Verification items for the finished model (mm, model axes). A direction names the side the tool comes from. Coordinates: 2 decimals unless noted, no trailing zeros. Write each loop counter-clockwise with the first axis right and the second up, starting at its lowest first coordinate (ties: lowest second). Pieces come first, ordered by that corner, then holes. Notation, with made-up numbers: (33, -20.75) - (77, -20.75) arc R20 cw to (77, 8.25) - close; hole circle Ø2 at (24, 40.5). An arc over 180 degrees is marked (long way). Use CSV: the item, a comma, the result in double quotes. Start each with the question number.
Autodesk Fusion 360 part; units mm, degrees
sketch "Sketch1" plane through (0, 0, 0) normal (0, 1, 0) x (1, 0, 0)
  line L0 (17.5, 25) -> (-17.5, 25)
  line L1 (-17.5, 25) -> (-17.5, -25)
  line L2 (-17.5, -25) -> (17.5, -25)
  line L3 (17.5, -25) -> (17.5, 25)
  line L4 (17.5, 25) -> (-17.5, -25) construction
  line L5 (-17.5, 25) -> (17.5, -25) construction
  line L6 (25, 17.5) -> (-25, 17.5)
  line L7 (-25, 17.5) -> (-25, -17.5)
  line L8 (-25, -17.5) -> (25, -17.5)
  line L9 (25, -17.5) -> (25, 17.5)
  line L10 (25, 17.5) -> (-25, -17.5) construction
  line L11 (-25, 17.5) -> (25, -17.5) construction
  circle A0 centre (0, 0) radius 7.6
  circle A1 centre (0, 0) radius 6.4
  circle A2 centre (0, 0) radius 12.5
  circle A3 centre (-20, 7.5) radius 1.5
  circle A4 centre (-20, -7.5) radius 1.5
  circle A5 centre (-7.5, -20) radius 1.5
  circle A6 centre (7.5, -20) radius 1.5
  circle A7 centre (20, -7.5) radius 1.5
  circle A8 centre (20, 7.5) radius 1.5
  circle A9 centre (7.5, 20) radius 1.5
  circle A10 centre (-7.5, 20) radius 1.5
  dimension "d1" = 50
  dimension "d2" = 35
  dimension "d3" = 50
  dimension "d4" = 35
  dimension "d5" = 15.2
  dimension "d6" = 12.8
  dimension "d7" = 25
  dimension "d8" = 3
  dimension "d9" = 3
  dimension "d10" = 10
  dimension "d11" = 10
  dimension "d12" = 5
  dimension "d13" = 5
  dimension "d15" = 360
extrude "Extrude1" add sketch "Sketch1" along normal blind 3 contours L0 L1 L3 L6 | L3 L6 L8 L9 | L1 L3 L6 L8 | L1 L6 L7 L8 | L1 L2 L3 L8 makes body 1
extrude "Extrude2" add sketch "Sketch1" along normal blind 10 separate body contours A0 makes body 2
extrude "Extrude3" add sketch "Sketch1" along normal blind 40 contours A1 | A2 bodies 1 2
sketch "Sketch2" plane through (0, 10, 0) normal (0, 1, 0) x (-1, 0, 0)
  circle A0 centre (0, 0) radius 6.4
  circle A1 centre (0, 0) radius 7.6
sketch "Sketch4" plane through (0, 0, 0) normal (0, 0, 1) x (1, 0, 0)
  circle A0 centre (0, 20) radius 1.5
  line L0 (0, 20) -> (0, 0)
  dimension "d22" = 3
  dimension "d23" = 20
extrude "Extrude4" cut sketch "Sketch4" against normal blind 30 bodies 1
extrude "Extrude5" cut sketch "Sketch4" along normal blind 30 bodies 1
sketch "Sketch6" plane through (0, 0, 0) normal (1, 0, 0) x (0, 0, -1)
  circle A0 centre (0, 30) radius 1.5
  line L0 (0, 30) -> (0, 0)
  dimension "d28" = 3
  dimension "d29" = 30
extrude "Extrude6" cut sketch "Sketch6" against normal blind 30 bodies 1
extrude "Extrude7" cut sketch "Sketch6" along normal blind 30 bodies 1
sketch "Sketch7" plane through (0, 0, 0) normal (0, 1, 0) x (1, 0, 0)
  circle A0 centre (0, 0) radius 1
  dimension "d34" = 2
extrude "Extrude8" cut sketch "Sketch7" along normal blind 10 bodies 1
Q1. Scan lines: line 1 along Z through (x, y) = (20, 1.1); line 2 along X through (y, z) = (1.55, 7.5). Record each from-to range of solid material in increasing order. Write a range as from..to.
Q2. Release check for a two-part mould opening along Z. For faces 1 (the cylindrical face through (-8.61, 1.48, 21.01)), 2 (the flat face through (-21, 1, -17.5)), 3 (the flat face through (-5.9, 3, -11.5)) record: released by +Z, released by -Z, zero draft, split by the parting line, or undercut.
Q3. Tool access check on faces 4 (the flat face through (-17.5, 1, 21)), 5 (the flat face through (0, 10, 0)), 6 (the cylindrical face through (6.104, 24.79, 1.922)), 7 (the flat face through (21, 1, -17.5)). Record the directions out of +Z, -Z, +X, -X, +Y, -Y that give a thin tool (end or side, any length) a straight path to the whole face; none if there is none.
Q4. Cross-section at C-C (y = 20). Record the cut outline in (x, z).
Q5. Cross-section at B-B (x = -20). Record the cut outline in (y, z).
Q6. Gauge pin test, flat ends, axial feed: pin 1 (2.5 mm diameter, centred on y = 30, z = 0, fed in from +X); pin 2 (10 mm diameter, centred on x = 5, y = 17, fed in from +Z); pin 3 (0.9 mm diameter, centred on x = 22.5, y = 1, fed in from -Z); pin 4 (3.5 mm diameter, centred on x = -21.5, y = 2, fed in from +Z). Record the tip position at first contact, or that the pin passes through.
Q7. Cross-section at A-A (z = 0). State how many separate pieces and enclosed holes the cut face has, plus the area to 3 significant figures.
Q8. Cross-section at D-D (y = 35.5). Record the cut outline in (x, z).
Reply:
1,line 1,"-17.5..-9, -6..6, 9..17.5"
1,line 2,"-25..-21.5, -18.5..18.5, 21.5..25"
2,face 1,"undercut"
2,face 2,"released by -Z"
2,face 3,"zero draft"
3,face 4,"+Z, -X, +Y, -Y"
3,face 5,"-Y"
3,face 6,"+Y"
3,face 7,"-Z, +X, +Y, -Y"
4,outline,"(-1.5, -12.41) - (-1.5, -7.45) arc R7.6 cw to (-1.5, 7.45) - (-1.5, 12.41) arc R12.5 ccw to start; (-1.5, -6.22) - (-1.5, 6.22) arc R6.4 ccw to start; (1.5, -12.41) arc R12.5 ccw to (1.5, 12.41) - (1.5, 7.45) arc R7.6 cw to (1.5, -7.45) - close; (1.5, -6.22) arc R6.4 ccw to (1.5, 6.22) - close"
5,outline,"(0, -17.5) - (3, -17.5) - (3, -9) - (0, -9) - close; (0, -6) - (3, -6) - (3, 6) - (0, 6) - close; (0, 9) - (3, 9) - (3, 17.5) - (0, 17.5) - close"
6,pin 1,"through"
6,pin 2,"z = 12.5"
6,pin 3,"z = -17.5"
6,pin 4,"z = 17.5"
7,separate pieces,"4"
7,enclosed holes,"1"
7,area,"908 mm^2"
8,outline,"circle Ø25 at (0, 0); circle Ø12.8 at (0, 0); hole circle Ø15.2 at (0, 0)"
